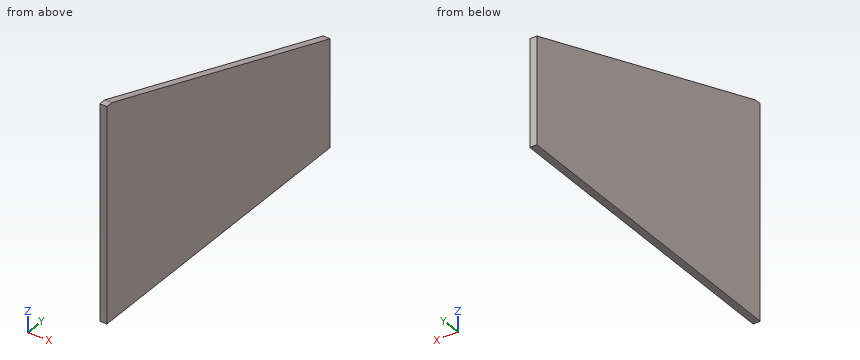
from build123d import *

# Parameters (mm, degrees)
F0_W     = 10
F0_H     = 300
F0_W_2   = 188.557307
F0_H_2   = 150
F1_DEPTH = 10


with BuildPart() as f1:
    # F0 (on Right) → F1 (new body)
    with BuildSketch(Plane.YZ):
        with Locations((-138.908036, 150)):
            Rectangle(F0_W, F0_H)
        Polygon((-133.908036, 300), (-133.908036, 0), (117.534657, 0), (117.534657, 150), (306.091964, 150), align=None)
        with Locations((211.81331, 75)):
            Rectangle(F0_W_2, F0_H_2)
    extrude(amount=F1_DEPTH)


solid = f1.part
The model under review builds one solid part; all positions refer to its coordinate system, in mm. Give positions to 0.01 mm unless a question says otherwise; leave off trailing zeros. Write each loop counter-clockwise with the first axis right and the second up, starting at its lowest first coordinate (ties: lowest second). Pieces come first, ordered by that corner, then holes.
1. Add section C-C, the plane y = 191. Write out the cut boundary in (x, z).
2. Add section B-B, the plane y = 104. Write out the cut boundary in (x, z), plus the area to 3 significant figures.
3. Wall thickness on L1, parallel to Z at x = 0.75, y = 278; L2, parallel to Z at x = 0.5, y = 206.5: over which ranges is each line inside the solid? List them lowest first.
4. Add section A-A, the plane x = 7.5. Write out the cut boundary in (y, z), plus the area to 3 significant figures.
Worked answers:
1. outline: (0, 0) - (10, 0) - (10, 189.24) - (0, 189.24) - close
2. outline: (0, 0) - (10, 0) - (10, 218.89) - (0, 218.89) - close
2. area: 2,190 mm2
3. L1: z = 0 to 159.58
3. L2: z = 0 to 183.95
4. outline: (-143.91, 0) - (306.09, 0) - (306.09, 150) - (-133.91, 300) - (-143.91, 300) - close
4. area: 102,000 mm2
